Here's how the part is built. I have some questions about the finished solid (model axes, mm). A direction names the side the tool comes from. Round coordinates to 2 decimals unless told otherwise and drop trailing zeros. Order: outer loops, then holes, each group sorted by start corner. A loop starts at its lowest first (then second) coordinate and runs counter-clockwise, first axis right, second up. Notation, with made-up numbers: (68.5, 40.25) - (82.5, 40.25) arc R13 ccw to (82.5, 53.25) - close; hole circle Ø3 at (10.5, -37.5). An arc over 180 degrees is marked (long way). One line per item, written item: value.
from build123d import *

# Parameters (mm, degrees)
SKETCH_1_W          = 34
SKETCH_1_H          = 34
EXTRUDE_1_DEPTH     = 8
SKETCH_2_W          = 24.5
SKETCH_2_H          = 24.5
CUT_EXTRUDE_1_DEPTH = 6
SKETCH_3_W          = 28.5
SKETCH_3_H          = 28.5
CUT_EXTRUDE_2_DEPTH = 3
SKETCH_4_W          = 12.5
SKETCH_4_H          = 12.5
EXTRUDE_2_DEPTH     = 6
SKETCH_5_W          = 34
SKETCH_5_H          = 34
SKETCH_5_W_2        = 28.5
SKETCH_5_H_2        = 28.5
SKETCH_5_W_3        = 12.5
SKETCH_5_H_3        = 12.5
CUT_EXTRUDE_4_DEPTH = 0.5


with BuildPart() as part:
    # Эскиз1 → Бобышка-Вытянуть1 (new body)
    with BuildSketch(Plane(origin=(0, 0, 0), x_dir=(1, 0, 0), z_dir=(0, 1, 0))):
        with Locations((17, 17)):
            Rectangle(SKETCH_1_W, SKETCH_1_H)
    extrude(amount=EXTRUDE_1_DEPTH)

    # Эскиз2 → Вырез-Вытянуть1 (cut)
    with BuildSketch(Plane(origin=(0, 8, 0), x_dir=(1, 0, 0), z_dir=(0, 1, 0))):
        with Locations((17, 17)):
            Rectangle(SKETCH_2_W, SKETCH_2_H)
    extrude(amount=-CUT_EXTRUDE_1_DEPTH, mode=Mode.SUBTRACT)

    # Эскиз3 → Вырез-Вытянуть2 (cut)
    with BuildSketch(Plane(origin=(0, 8, 0), x_dir=(1, 0, 0), z_dir=(0, 1, 0))):
        with Locations((17, 17)):
            Rectangle(SKETCH_3_W, SKETCH_3_H)
    extrude(amount=-CUT_EXTRUDE_2_DEPTH, mode=Mode.SUBTRACT)

    # Эскиз4 → Бобышка-Вытянуть2 (add)
    with BuildSketch(Plane(origin=(0, 2, 0), x_dir=(1, 0, 0), z_dir=(0, 1, 0))):
        with Locations((17, 17)):
            Rectangle(SKETCH_4_W, SKETCH_4_H)
    extrude(amount=EXTRUDE_2_DEPTH)

    # Эскиз5 → Вырез-Вытянуть4 (cut)
    # profile 1 of 2: a face of its own
    with BuildSketch(Plane(origin=(0, 8, 0), x_dir=(1, 0, 0), z_dir=(0, 1, 0))):
        with Locations((17, 17)):
            Rectangle(SKETCH_5_W, SKETCH_5_H)
        with Locations((17, 17)):
            Rectangle(SKETCH_5_W_2, SKETCH_5_H_2, mode=Mode.SUBTRACT)
    # profile 2 of 2: a face of its own
    with BuildSketch(Plane(origin=(0, 8, 0), x_dir=(1, 0, 0), z_dir=(0, 1, 0))):
        with Locations((17, 17)):
            Rectangle(SKETCH_5_W_3, SKETCH_5_H_3)
    extrude(amount=-CUT_EXTRUDE_4_DEPTH, mode=Mode.SUBTRACT)


solid = part.part
Q1. We'd pull the mould along X, two halves only. Please class faces 3 (the flat face through (0, 4, -17)), 4 (the flat face through (10.75, 5, -17)), 5 (the flat face through (2, 7.5, -17)): released by +X, released by -X, zero draft, split by the parting line, or undercut.
Results list:
face 3: released by -X
face 4: undercut
face 5: zero draft
Q2. If we section it at B-B, the plane x = 3.5: Please give me the cut outline in (y, z).
Results list:
outline: (0, -34) - (7.5, -34) - (7.5, -31.25) - (5, -31.25) - (5, -2.75) - (7.5, -2.75) - (7.5, 0) - (0, 0) - close
Q3. If we section it at A-A, the plane y = 7: Please give me the cut outline in (x, z).
Results list:
outline: (0, -34) - (34, -34) - (34, 0) - (0, 0) - close; (10.75, -23.25) - (23.25, -23.25) - (23.25, -10.75) - (10.75, -10.75) - close; hole (2.75, -31.25) - (31.25, -31.25) - (31.25, -2.75) - (2.75, -2.75) - close
Q4. Will this pin go through, and if not, where does the flat tip stop? pin 1 (1 mm diameter, centred on x = 17, z = -7, fed in from +Y).
Results list:
pin 1: y = 2
Q5. If we section it at C-C, the plane z = -13: Please give me the cut outline in (x, y), then the cut area to 3 significant figures.
Results list:
outline: (0, 0) - (34, 0) - (34, 7.5) - (31.25, 7.5) - (31.25, 5) - (29.25, 5) - (29.25, 2) - (23.25, 2) - (23.25, 7.5) - (10.75, 7.5) - (10.75, 2) - (4.75, 2) - (4.75, 5) - (2.75, 5) - (2.75, 7.5) - (0, 7.5) - close
area: 179 mm²
Q6. If we section it at D-D, the plane y = 4: Please give me the cut outline in (x, z), then the cut area to 3 significant figures.
Results list:
outline: (0, -34) - (34, -34) - (34, 0) - (0, 0) - close; (10.75, -23.25) - (23.25, -23.25) - (23.25, -10.75) - (10.75, -10.75) - close; hole (4.75, -29.25) - (29.25, -29.25) - (29.25, -4.75) - (4.75, -4.75) - close
area: 712 mm²
Q7. If I drill on line 1 along Z through (x, y) = (17, 4.25); line 2 along X through (y, z) = (4.25, -23); line 3 along Z through (x, y) = (22.5, 6), over which ranges is the centre line in solid material (lowest first)?
Results list:
line 1: -34 to -29.25, -23.25 to -10.75, -4.75 to 0
line 2: 0 to 4.75, 10.75 to 23.25, 29.25 to 34
line 3: -34 to -31.25, -23.25 to -10.75, -2.75 to 0
Q8. Which directions (+Z, -Z, +X, -X, +Y, -Y) give clear straight access to the entire face, cutting with the end or side of a thin tool? Please do faces 1 (the flat face through (17, 4, 0)), 2 (the flat face through (17, 4, -4.75)).
Results list:
face 1: +Z, +X, -X, +Y, -Y
face 2: +Y
